Read the model definition and answer for the solid it produces. Units are mm, in the model's axes. A direction names the side the tool comes from. Give positions to 0.01 mm unless a question says otherwise; leave off trailing zeros. Loops run counter-clockwise (first coordinate to the right, second up) from the corner with the lowest first, then second, coordinate; pieces in that order, holes last. Notation, with made-up numbers: (-3.75, 66) -> (10.25, 66) arc R14 cw to (10.25, 71) -> close; hole circle Ø8 at (5.25, 18). An arc over 180 degrees is marked (long way). Write each question's results on one line, items separated by ' | '. Start each with the question number.
Item 1: Determine the mould class of faces 4 (the cylindrical face through (113.147, -14.77, 6.465)), 5 (the flat face through (-22, -22, 47)), 6 (the flat face through (123, 21, 4)), 7 (the cylindrical face through (8.362, 6.654, 46.744)) for opening direction Y: +Y half, -Y half, draft (parallel to the pull), parting line (faces both ways), or undercut.
Item 2: Section D-D on x = 29 is taken. Write down the section's boundary in (y, z), and give its area (3 significant figures).
Item 3: Section A-A on x = -8.85 is taken. Write down the section's boundary in (y, z), and give its area (3 significant figures).
Item 4: Each of these flat-tipped pins is pushed along its axis until it touches: P1, Ø14.5, axis at x = 81, y = 10.5, coming from the +Z side; P2, Ø4, axis at x = 114.845, y = -14.845, coming from the -Z side; P3, Ø5, axis at y = -17.5, z = 13, coming from the -X side. Where does it stop, or does it pass through?
Item 5: Which of the six approach directions +Z, -Z, +X, -X, +Y, -Y give full straight-line access (tool end or side, diameter ignored) to faces 1 (the flat face through (-8, 5, 47)), 2 (the flat face through (11, 0, 42.8)), 3 (the cylindrical face through (118.31, 13.41, 1.97))?
Item 6: Find the intervals of material crossed by line 1 (Y direction, x = 8.85, z = 47.5); line 2 (X direction, y = 8, z = 48); line 3 (Z direction, x = 72.5, y = 14), in increasing order.
Item 7: Section B-B on y = 8.85 is taken. Write down the section's boundary in (x, z).
Item 8: Section C-C on z = 25.5 is taken. Write down the section's boundary in (x, y).
```python
from build123d import *

# Parameters (mm, degrees)
SKETCH_1_R        = 3.75
EXTRUDE_244_DEPTH = 4
EXTRUDE_START     = 4
SKETCH_2_R        = 1.7
EXTRUDE_328_DEPTH = 5
EXTRUDE_START_2   = 9
SKETCH_3_W        = 13
SKETCH_3_H        = 48
EXTRUDE_401_DEPTH = 33.8
EXTRUDE_START_3   = 42.8
SKETCH_4_R        = 2.25
EXTRUDE_499_DEPTH = 8


with BuildPart() as part:
    # 草图1 → Extrude 244 (new body)
    with BuildSketch(Plane.XY):
        Polygon((48, -24), (120, -24), (125, -19), (125, 19), (120, 24), (48, 24), align=None)
        with Locations((85.155, -14.845)):
            Circle(SKETCH_1_R, mode=Mode.SUBTRACT)
        with Locations((85.155, 14.845)):
            Circle(SKETCH_1_R, mode=Mode.SUBTRACT)
        with Locations((114.845, -14.845)):
            Circle(SKETCH_1_R, mode=Mode.SUBTRACT)
        with Locations((114.845, 14.845)):
            Circle(SKETCH_1_R, mode=Mode.SUBTRACT)
    extrude(amount=EXTRUDE_244_DEPTH)

    # 草图2 → Extrude 328 (add)
    with BuildSketch(Plane.XY.offset(EXTRUDE_START)):
        Polygon((48, -24), (120, -24), (125, -19), (125, 19), (120, 24), (48, 24), align=None)
        with Locations((85.155, -14.845)):
            Circle(SKETCH_2_R, mode=Mode.SUBTRACT)
        with Locations((85.155, 14.845)):
            Circle(SKETCH_2_R, mode=Mode.SUBTRACT)
        with Locations((114.845, -14.845)):
            Circle(SKETCH_2_R, mode=Mode.SUBTRACT)
        with Locations((114.845, 14.845)):
            Circle(SKETCH_2_R, mode=Mode.SUBTRACT)
    extrude(amount=EXTRUDE_328_DEPTH)

    # 草图3 → Extrude 401 (add)
    with BuildSketch(Plane.XY.offset(EXTRUDE_START_2)):
        with Locations((54.5, 0)):
            Rectangle(SKETCH_3_W, SKETCH_3_H)
    extrude(amount=EXTRUDE_401_DEPTH)

    # 草图4 → Extrude 499 (add)
    with BuildSketch(Plane.XY.offset(EXTRUDE_START_3)):
        Polygon((-24, -20), (-20, -24), (61, -24), (61, 24), (-20, 24), (-24, 20), (-24, 5), (8, 5), (8, -5), (-24, -5), align=None)
        with Locations((-8.85, -8.85)):
            Circle(SKETCH_4_R, mode=Mode.SUBTRACT)
        with Locations((-8.85, 8.85)):
            Circle(SKETCH_4_R, mode=Mode.SUBTRACT)
        with Locations((8.85, -8.85)):
            Circle(SKETCH_4_R, mode=Mode.SUBTRACT)
        with Locations((8.85, 8.85)):
            Circle(SKETCH_4_R, mode=Mode.SUBTRACT)
    extrude(amount=EXTRUDE_499_DEPTH)


solid = part.part
```
Findings:
1) face 4: undercut | face 5: -Y half | face 6: +Y half | face 7: undercut
2) outline: (-24, 42.8) -> (24, 42.8) -> (24, 50.8) -> (-24, 50.8) -> close | area: 384 mm2
3) outline: (-24, 42.8) -> (-11.1, 42.8) -> (-11.1, 50.8) -> (-24, 50.8) -> close; (-6.6, 42.8) -> (-5, 42.8) -> (-5, 50.8) -> (-6.6, 50.8) -> close; (5, 42.8) -> (6.6, 42.8) -> (6.6, 50.8) -> (5, 50.8) -> close; (11.1, 42.8) -> (24, 42.8) -> (24, 50.8) -> (11.1, 50.8) -> close | area: 232 mm2
4) P1: z = 9 | P2: z = 4 | P3: x = 48
5) face 1: +Z, -Z, -X | face 2: -Z, -X, +Y, -Y | face 3: -Z
6) line 1: -24 to -11.1, -6.6 to 6.6, 11.1 to 24 | line 2: -24 to -10.93, -6.77 to 6.77, 10.93 to 61 | line 3: 0 to 9
7) outline: (-24, 42.8) -> (-11.1, 42.8) -> (-11.1, 50.8) -> (-24, 50.8) -> close; (-6.6, 42.8) -> (6.6, 42.8) -> (6.6, 50.8) -> (-6.6, 50.8) -> close; (11.1, 42.8) -> (48, 42.8) -> (48, 0) -> (125, 0) -> (125, 9) -> (61, 9) -> (61, 50.8) -> (11.1, 50.8) -> close
8) outline: (48, -24) -> (61, -24) -> (61, 24) -> (48, 24) -> close
